```python
from build123d import *

# Parameters (mm, degrees)
SWEEP1_START        = -19.05
SWEEP1_DEPTH        = 38.1
BOSS_EXTRUDE1_START = -9.525
SKETCH4_R           = 3.175
BOSS_EXTRUDE1_DEPTH = 19.05
FILLET1_R           = 12.7


# Read off the part's stored shape, not the designer's step: Sweep1
with BuildPart() as part:
    # Sweep1 outline → Sweep1 (new body)
    with BuildSketch(Plane.XY.offset(SWEEP1_START)):
        Polygon((101.6, 41.275), (101.6, 60.325), (50.8, 60.325), (0, 9.525), (0, -9.525), (50.8, 41.275), align=None)
    extrude(amount=SWEEP1_DEPTH)

    # Sketch4 → Boss-Extrude1 (add)
    with BuildSketch(Plane(origin=(0, 0, 0), x_dir=(1, 0, 0), z_dir=(0, 1, 0)).offset(BOSS_EXTRUDE1_START)):
        with BuildLine():
            Line((0, 19.05), (-12.7, 19.05))
            ThreePointArc((-12.7, 19.05), (-31.75, 0), (-12.7, -19.05))
            Line((-12.7, -19.05), (0, -19.05))
            Line((0, -19.05), (0, 19.05))
        make_face()
        with Locations(Location((-12.7, 0, 0), (0, 0, 90))):
            Circle(SKETCH4_R, mode=Mode.SUBTRACT)
    extrude(amount=BOSS_EXTRUDE1_DEPTH)

    # Mirror4: part across plane


with BuildPart() as part_1:
    add(part.part)
    add(part.part.mirror(Plane(origin=(101.6, 0, 0), x_dir=(0, 0, 1), z_dir=(1, 0, 0))))

    # Fillet1
    fillet1_edges = [part_1.edges().sort_by_distance(p)[0] for p in [
        (50.8, 60.325, 0),
        (50.8, 41.275, 0),
        (152.4, 60.325, 0),
        (152.4, 41.275, 0),
    ]]
    fillet(fillet1_edges, radius=FILLET1_R)


solid = part_1.part
```
The listing builds one solid part. Answer for the finished solid, in the listing's coordinates (mm). A direction names the side the tool comes from. Give positions to 0.01 mm unless a question says otherwise; leave off trailing zeros. Write each loop counter-clockwise with the first axis right and the second up, starting at its lowest first coordinate (ties: lowest second). Pieces come first, ordered by that corner, then holes. Notation, with made-up numbers: M 28.25,-6 L 40.25,-6 A27 ccw 40.25,25 Z; hole C 37,-2 d7. An arc over 180 degrees is marked long. Write each question's results on one line, items separated by ' | '.
Q1. Section B-B, the plane z = 0 is taken. Write down the section's boundary in (x, y) (3 decimals), then the cut area to 3 significant figures.
Output values:
outline: M -31.75,-9.525 L -15.875,-9.525 L -15.875,9.525 L -31.75,9.525 Z; M -9.525,-9.525 L 0,-9.525 L 47.08,37.555 A12.7 cw 56.061,41.275 L 147.139,41.275 A12.7 cw 156.12,37.555 L 203.2,-9.525 L 212.725,-9.525 L 212.725,9.525 L 203.2,9.525 L 156.12,56.605 A12.7 ccw 147.139,60.325 L 56.061,60.325 A12.7 ccw 47.08,56.605 L 0,9.525 L -9.525,9.525 Z; M 219.075,-9.525 L 234.95,-9.525 L 234.95,9.525 L 219.075,9.525 Z | area: 4,840 mm2
Q2. Consider L1, parallel to X at y = 2.75, z = 0 (3 decimals); L2, parallel to X at y = -4, z = 0 (3 decimals); L3, parallel to Z at x = 215.9, y = 1 (3 decimals). Determine where each line is inside the solid, lowest interval first. Write a range as from..to.
Output values:
L1: -31.75..-15.875, -9.525..12.275, 190.925..212.725, 219.075..234.95 | L2: -31.75..-15.875, -9.525..5.525, 197.675..212.725, 219.075..234.95 | L3: -19.05..-3.175, 3.175..19.05
Q3. Section C-C, the plane y = 15 is taken. Write down the section's boundary in (x, z) (3 decimals).
Output values:
outline: M 5.475,-19.05 L 24.525,-19.05 L 24.525,19.05 L 5.475,19.05 Z; M 178.675,-19.05 L 197.725,-19.05 L 197.725,19.05 L 178.675,19.05 Z
Q4. For a pull along Z with two mould halves and no side action, classify faces 1 (the cylindrical face through (212.8, -0.13, 0.69)), 2 (the flat face through (23.87, 33.395, -0.267)), 3 (the cylindrical face through (-31.745, -0.133, -0.419)) as released by +Z, released by -Z, zero draft, split by the parting line, or undercut.
Output values:
face 1: undercut | face 2: zero draft | face 3: split by the parting line
Q5. Flat-ended cylindrical pins translate along their axes: P1, Ø5, axis at x = 115, z = 10, coming from the -Y side (3 decimals); P2, Ø1.5, axis at y = 20.5, z = -14.5, coming from the +X side (3 decimals); P3, Ø2, axis at y = 18, z = -4, coming from the +X side (3 decimals); P4, Ø5, axis at x = -12.7, z = 0, coming from the +Y side. Find the tip coordinate at first contact, or state that the pin passes through.
Output values:
P1: y = 41.275 | P2: x = 192.975 | P3: x = 195.725 | P4: through
Q6. A tool of negligible diameter and unlimited length cuts with its end or side. For faces 4 (the flat face through (219.3, 9.525, -0.3)), 5 (the flat face through (102, 41.275, 0)), 6 (the flat face through (-16.1, 9.525, -0.3)), 7 (the flat face through (219.3, -9.525, -0.3)), from which of +Z, -Z, +X, -X, +Y, -Y can it reach the whole face along a straight path? Write none if from no direction.
Output values:
face 4: +Z, -Z, +X, +Y | face 5: +Z, -Z, -Y | face 6: +Z, -Z, -X, +Y | face 7: +Z, -Z, +X, -X, -Y
Q7. Section A-A, the plane y = -3 is taken. Write down the section's boundary in (x, z) (3 decimals).
Output values:
outline: M -12.7,-19.05 L 6.525,-19.05 L 6.525,19.05 L -12.7,19.05 A19.05 ccw Z; M 196.675,-19.05 L 215.9,-19.05 A19.05 ccw 215.9,19.05 L 196.675,19.05 Z; hole C -12.7,0 d6.35; hole C 215.9,0 d6.35
Q8. Section D-D, the plane x = 68.5 is taken. Write down the section's boundary in (y, z) (3 decimals), then the cut area to 3 significant figures.
Output values:
outline: M 41.275,-19.05 L 60.325,-19.05 L 60.325,19.05 L 41.275,19.05 Z | area: 726 mm2
